Here's how the part is built. I have some questions about the finished solid (model axes, mm). Round coordinates to 2 decimals unless told otherwise and drop trailing zeros. Loops run counter-clockwise (first coordinate to the right, second up) from the corner with the lowest first, then second, coordinate; pieces in that order, holes last. Notation, with made-up numbers: (51, 56) - (95, 56) arc R29 ccw to (95, 77) - close; hole circle Ø3 at (43.5, -16.5). An arc over 180 degrees is marked (long way). Answer as a JSON object with one key per item and string values. Group by question number.
1) I want a section at A-A, the plane x = 0. Please give me the cut outline in (y, z), then the cut area to 4 significant figures.
2) I want a section at B-B, the plane z = 105. Please give me the cut outline in (x, y).
3) Will these pins go through, and if not, where does the flat tip stop? P1, Ø6, axis at x = 8.5, y = -4, coming from the -Z side; P2, Ø1.2, axis at x = 3.5, z = -143, coming from the -Y side; P3, Ø1.6, axis at x = -4, z = -143.5, coming from the +Y side; P4, Ø1.5, axis at y = 12.5, z = 66.5, coming from the -X side.
4) I want a section at C-C, the plane x = -13. Please give me the cut outline in (y, z), then the cut area to 3 significant figures.
5) If I drill on line 1 along Z through (x, y) = (-4, 0); line 2 along Z through (x, y) = (7.5, -11.5); line 3 along Y through (x, z) = (0.5, -7.5), over which ranges is the centre line in solid material (lowest first)? Write a range as [from, to].
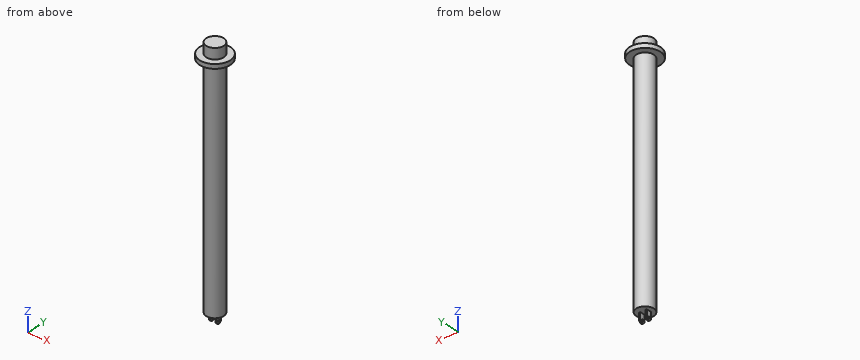
Autodesk Inventor part; units mm, degrees
ref_plane "YZ Plane" through (0, 0, 0) normal (1, 0, 0) x (0, 1, 0)
ref_plane "XZ Plane" through (0, 0, 0) normal (0, 1, 0) x (-1, 0, 0)
ref_plane "XY Plane" through (0, 0, 0) normal (0, 0, 1) x (1, 0, 0)
sketch "草图1" plane through (0, 0, 0) normal (0, 0, 1) x (1, 0, 0)
  circle A0 centre (0, 0) radius 10
  dimension "d0" = 20
extrude "拉伸1" add sketch "草图1" along normal mid plane 280
sketch "草图2" plane through (0, 0, -140) normal (0, 0, -1) x (-1, 0, 0)
  line L0 (-4.5, 3) -> (-3, 3)
  line L1 (-3, 3) -> (-3, -3)
  line L2 (-3, -3) -> (-4.5, -3)
  line L3 (-4.5, -3) -> (-4.5, 3)
  line L4 (0, 0) -> (0, 6.2448)
  line L5 (4.5, 3) -> (3, 3)
  line L6 (3, 3) -> (3, -3)
  line L7 (3, -3) -> (4.5, -3)
  line L8 (4.5, -3) -> (4.5, 3)
  point P0 (-3, 0)
  point P1 (3, 0)
  dimension "d3" = 1.5
  dimension "d4" = 6
  dimension "d5" = 6
extrude "拉伸2" add sketch "草图2" along normal blind 10
full round fillet "全圆角1" first side at (4, -3, -143.3333) centre faces at (4, 1, -150) second side at (3.5, 3, -143.3333)
full round fillet "全圆角2" first side at (-3.5, -3, -143.3333) centre faces at (-3.5, 1, -150) second side at (-4, 3, -143.3333)
sketch "草图3" plane through (-4.5, -3, -140) normal (-1, 0, 0) x (0, 0, 1)
  arc A0 (-7, 6) -> (-7, 0) centre (-7, 3) ccw
  point P0 (140, 3)
hole "孔1" at (-4.5, 0, -147) direction (1, 0, 0) diameter 2 end through all
ref_plane "工作平面1" through (0, 0, 123) normal (0, 0, 1) x (1, 0, 0)
sketch "草图4" plane through (0, 0, 123) normal (0, 0, 1) x (1, 0, 0)
  circle A0 centre (0, 0) radius 17.5
  dimension "d16" = 35
extrude "拉伸3" add sketch "草图4" along normal blind 5
properties part number "顶杆"
Outcome:
{
 "1": {"outline": "(-17.5, 123) - (-10, 123) - (-10, -140) - (10, -140) - (10, 123) - (17.5, 123) - (17.5, 128) - (10, 128) - (10, 140) - (-10, 140) - (-10, 128) - (-17.5, 128) - close", "area": "5,675 mm^2"},
 "2": {"outline": "circle Ø20 at (0, 0)"},
 "3": {"P1": "z = -140", "P2": "y = -3", "P3": "y = 3", "P4": "through"},
 "4": {"outline": "(-11.72, 123) - (11.72, 123) - (11.72, 128) - (-11.72, 128) - close", "area": "117 mm^2"},
 "5": {"line 1": "[-150, -148], [-146, 140]", "line 2": "[123, 128]", "line 3": "[-9.99, 9.99]"}
}
